Read the model definition and answer for the solid it produces. Units are mm, in the model's axes. Face numbers are marked on the shaded views. A direction names the side the tool comes from. Coordinates: 2 decimals unless noted, no trailing zeros. Order: outer loops, then holes, each group sorted by start corner. A loop starts at its lowest first (then second) coordinate and runs counter-clockwise, first axis right, second up. Notation, with made-up numbers: M 25.5,61 L 62.5,61 A14 cw 62.5,83 Z; hole C -37.5,75.5 d3. An arc over 180 degrees is marked long. Write each question's results on one line, items separated by ' | '.
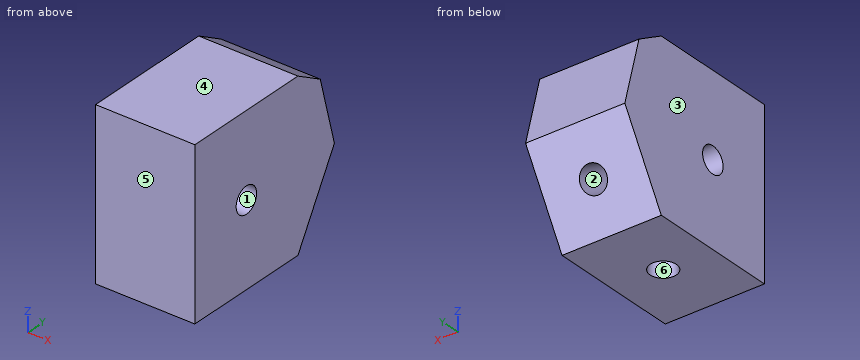
```python
from build123d import *

# Parameters (mm, degrees)
ESBO_O1_R                = 3.97
RESSALTO_EXTRUS_O1_DEPTH = 15
ESBO_O3_R                = 3.97
CORTE_EXTRUS_O2_DEPTH    = 25
CHANFRO1_SIZE            = 15
ESBO_O4_R                = 3.97
CORTE_EXTRUS_O3_DEPTH    = 15


with BuildPart() as part:
    # Esboço1 → Ressalto-extrusão1 (new body, symmetric)
    with BuildSketch(Plane(origin=(0, 0, 0), x_dir=(0, 0, -1), z_dir=(1, 0, 0))):
        Polygon((25, -20), (-25, -20), (-25, 20), (-12.5, 41.650635095), (25, 20), align=None)
        Circle(ESBO_O1_R, mode=Mode.SUBTRACT)
    extrude(amount=RESSALTO_EXTRUS_O1_DEPTH, both=True)

    # Esboço3 → Corte-extrusão2 (cut)
    with BuildSketch(Plane(origin=(0, 0, -25), x_dir=(-1, 0, 0), z_dir=(0, 0, -1))):
        Circle(ESBO_O3_R)
    extrude(amount=-CORTE_EXTRUS_O2_DEPTH, mode=Mode.SUBTRACT)

    # Chanfro1
    chanfro1_edges = [part.edges().sort_by_distance(p)[0] for p in [
        (0, 41.650635095, 12.5),
    ]]
    chamfer(chanfro1_edges, length=CHANFRO1_SIZE)

    # Esboço4 → Corte-extrusão3 (cut)
    with BuildSketch(Plane(origin=(0, 25.825317547, -14.910254038), x_dir=(1, 0, 0), z_dir=(0, 0.866025404, -0.5))):
        with Locations((0, -2.5)):
            Circle(ESBO_O4_R)
    extrude(amount=-CORTE_EXTRUS_O3_DEPTH, mode=Mode.SUBTRACT)


solid = part.part
```
(1) The part is cut by section D-D, the plane z = 18. Write down the section's boundary in (x, y).
Conclusion:
outline: M -15,-20 L 15,-20 L 15,29.2 L -15,29.2 Z
(2) Straight lines are drawn through the part: line 1 (Y direction, x = 0, z = -13.25); line 2 (X direction, y = 0, z = -17); line 3 (Y direction, x = -7.5, z = 20). For each, find the intervals that lie inside material, in ascending order.
Conclusion:
line 1: -20 to -3.97, 3.97 to 20.01 | line 2: -15 to -3.97, 3.97 to 15 | line 3: -20 to 28.66
(3) The mould has two halves that part along Z. Classify the marked faces 1, 2, 3 and 4: pulls with the +Z half, pulls with the -Z half, needs draft (parallel to the pull), parting line crosses it, or undercut.
Conclusion:
face 1: undercut | face 2: undercut | face 3: needs draft | face 4: pulls with the +Z half
(4) The part is cut by section B-B, the plane x = 0. Write down the section's boundary in (y, z).
Conclusion:
outline: M -20,-25 L -3.97,-25 L -3.97,0 A3.97 cw 3.97,0 L 3.97,-25 L 20,-25 L 25.09,-16.18 L 12.1,-8.68 L 16.07,-1.81 L 29.06,-9.31 L 34.15,-0.49 L 28.66,20 L 20,25 L -20,25 Z
(5) For the marked faces 5 and 6, determine the directions among +Z, -Z, +X, -X, +Y, -Y from which every point of the face is accessible in a straight line to the end or side of a thin tool.
Conclusion:
face 5: +Z, -Z, +X, -X, -Y | face 6: -Z
(6) The part is cut by section C-C, the plane z = 10.5. Write down the section's boundary in (x, y).
Conclusion:
outline: M -15,-20 L 15,-20 L 15,31.21 L -15,31.21 Z
(7) Given pin 1 (6.5 mm diameter, centred on y = 0, z = 0, fed in from -X); pin 2 (1 mm diameter, centred on x = -3.5, z = -18, fed in from +Y); pin 3 (12 mm diameter, centred on x = 2.5, z = 19, fed in from +Y), each flat-ended and moving along its own axis, determine where each tip first touches the part or whether it passes through.
Conclusion:
pin 1: through | pin 2: y = 24.33 | pin 3: y = 30.54
(8) The part is cut by section A-A, the plane x = -6. Write down the section's boundary in (y, z).
Conclusion:
outline: M -20,-25 L 20,-25 L 34.15,-0.49 L 28.66,20 L 20,25 L -20,25 Z; hole C 0,0 d7.94
